Source: CAD feature listing. Evaluate the final solid. Frame: model axes, mm. Face numbers are marked on the shaded views. A direction names the side the tool comes from. Coordinates: 2 decimals unless noted, no trailing zeros. Write each loop counter-clockwise with the first axis right and the second up, starting at its lowest first coordinate (ties: lowest second). Pieces come first, ordered by that corner, then holes. Notation, with made-up numbers: M 72,-5.5 L 83,-5.5 A14 ccw 83,2.5 Z; hole C 74.5,59 d7. An arc over 180 degrees is marked long. Write item = value, one per line. Start each with the question number.
1. Pull-direction query (X, two-part tool) for the marked faces 1, 2, 3 and 4; classes: pulls with the +X half, pulls with the -X half, needs draft (parallel to the pull), parting line crosses it, or undercut.
2. Access query for the marked faces 5, 6 and 7. Directions: +Z, -Z, +X, -X, +Y, -Y. A direction counts if a zero-diameter tool reaches every point of the face in a straight line with its end or side. Return the directions, or none.
3. Section query C-C (y = 5.5). Output: boundary loops of the cut face in (x, z).
4. Line query: line 1 along Z through (x, y) = (7.2, 0.3); line 2 along Z through (x, y) = (-7.2, 0.45); line 3 along X through (y, z) = (8.25, 10). Output: solid intervals per line, ascending.
5. Pin query (flat end, axial travel): pin 1 Ø6 at (x, z) = (-5.5, 11) entering from +Y; pin 2 Ø4.5 at (x, z) = (7.2, 30.8) entering from -Y; pin 3 Ø5.5 at (x, z) = (-5.5, 15) entering from +Y; pin 4 Ø6 at (y, z) = (9, 22) entering from -X. Return the tip coordinate at first contact, or that it passes through.
6. Section query D-D (x = 7.2). Output: boundary loops of the cut face in (y, z), then the cut area to 3 significant figures.
7. Section query A-A (z = 30.8). Output: boundary loops of the cut face in (x, y).
8. Section query B-B (x = -7.2). Output: boundary loops of the cut face in (y, z).
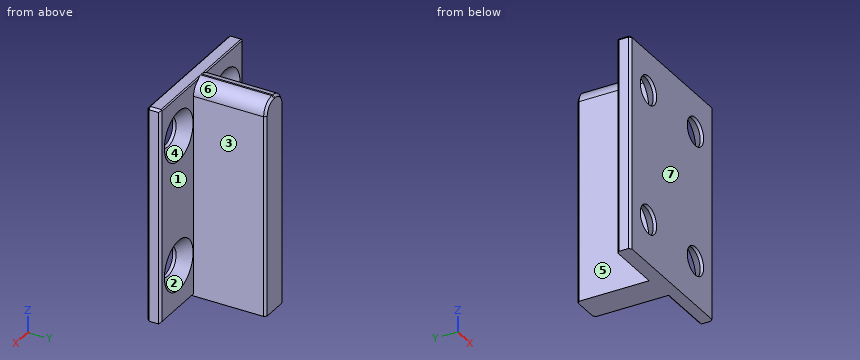
```python
from build123d import *

# Parameters (mm, degrees)
F1_DEPTH = 38
F2_R     = 2.5
F3_DEPTH = 25
F4_SIZE  = 1.9
F5_R     = 2.5
F6_SIZE  = 0.4
F7_SIZE  = 0.2


with BuildPart() as f1:
    # F0 (on Top) → F1 (new body)
    with BuildSketch(Plane.XY):
        Polygon((2.65, 15.3), (0, 15.3), (-2.65, 15.3), (-2.65, 2.5), (-12.65, 2.5), (-12.65, 0), (0, 0), (12.65, 0), (12.65, 2.5), (2.65, 2.5), align=None)
    extrude(amount=F1_DEPTH)

    # F2 (on Front) → F3 (cut)
    with BuildSketch(Plane.XZ):
        with Locations((-7.2, 30.8)):
            Circle(F2_R)
        with Locations((-7.2, 7.8)):
            Circle(F2_R)
        with Locations((7.2, 7.8)):
            Circle(F2_R)
        with Locations((7.2, 30.8)):
            Circle(F2_R)
    extrude(amount=-F3_DEPTH, mode=Mode.SUBTRACT)

    # F4
    f4_edges = [f1.edges().sort_by_distance(p)[0] for p in [
        (4.7, 2.5, 7.8),
        (4.7, 2.5, 30.8),
        (-9.7, 2.5, 7.8),
        (-9.7, 2.5, 30.8),
    ]]
    chamfer(f4_edges, length=F4_SIZE)

    # F5
    f5_edges = [f1.edges().sort_by_distance(p)[0] for p in [
        (-2.65, 8.9, 38),
        (2.65, 8.9, 38),
    ]]
    fillet(f5_edges, radius=F5_R)

    # F6
    f6_edges = [f1.edges().sort_by_distance(p)[0] for p in [
        (-2.65, 15.3, 17.75),
        (2.65, 15.3, 17.75),
        (7.65, 2.5, 0),
        (12.65, 2.5, 19),
        (0, 0, 38),
        (12.65, 0, 19),
        (-12.65, 2.5, 19),
        (-12.65, 0, 19),
        (-12.65, 1.25, 38),
        (12.65, 1.25, 38),
    ]]
    chamfer(f6_edges, length=F6_SIZE)

    # F7
    f7_edges = [f1.edges().sort_by_distance(p)[0] for p in [
        (7.45, 2.5, 38),
        (-7.45, 2.5, 38),
    ]]
    chamfer(f7_edges, length=F7_SIZE)


solid = f1.part
```
Results are:
q1.face_1 = needs draft
q1.face_2 = undercut
q1.face_3 = pulls with the +X half
q1.face_4 = undercut
q2.face_5 = +Z, -Z, -X, +Y
q2.face_6 = +Z, +X, +Y
q2.face_7 = +Z, -Z, +X, -X, -Y
q3.outline = M -2.65,0 L 2.65,0 L 2.65,35.5 A2.5 ccw 0.15,38 L -0.15,38 A2.5 ccw -2.65,35.5 Z
q4.line_1 = 0 to 5.3, 10.3 to 28.3, 33.3 to 37.9
q4.line_2 = 0 to 5.3, 10.3 to 28.3, 33.3 to 38
q4.line_3 = -2.65 to 2.65
q5.pin_1 = 15.05
q5.pin_2 = through
q5.pin_3 = 2.5
q5.pin_4 = -2.65
q6.outline = M 0,0 L 2.1,0 L 2.5,0.4 L 2.5,3.4 L 0.6,5.3 L 0,5.3 Z; M 0,10.3 L 0.6,10.3 L 2.5,12.2 L 2.5,26.4 L 0.6,28.3 L 0,28.3 Z; M 0,33.3 L 0.6,33.3 L 2.5,35.2 L 2.5,37.8 L 2.3,38 L 0.4,38 L 0,37.6 Z
q6.area = 62.6 mm^2
q7.outline = M -12.65,0.4 L -12.25,0 L -9.7,0 L -9.7,0.6 L -11.6,2.5 L -12.25,2.5 L -12.65,2.1 Z; M -4.7,0 L 4.7,0 L 4.7,0.6 L 2.8,2.5 L 2.65,2.5 L 2.65,14.9 L 2.25,15.3 L -2.25,15.3 L -2.65,14.9 L -2.65,2.5 L -2.8,2.5 L -4.7,0.6 Z; M 9.7,0 L 12.25,0 L 12.65,0.4 L 12.65,2.1 L 12.25,2.5 L 11.6,2.5 L 9.7,0.6 Z
q8.outline = M 0,0 L 2.5,0 L 2.5,3.4 L 0.6,5.3 L 0,5.3 Z; M 0,10.3 L 0.6,10.3 L 2.5,12.2 L 2.5,26.4 L 0.6,28.3 L 0,28.3 Z; M 0,33.3 L 0.6,33.3 L 2.5,35.2 L 2.5,37.8 L 2.3,38 L 0.4,38 L 0,37.6 Z
